CAD build for the part. Positions are in the model's coordinates, mm. Round coordinates to 2 decimals unless told otherwise and drop trailing zeros. Order: outer loops, then holes, each group sorted by start corner. A loop starts at its lowest first (then second) coordinate and runs counter-clockwise, first axis right, second up. Notation, with made-up numbers: (-32, -19) - (10, -19) arc R19 cw to (10, 14) - close; hole circle Ø3 at (6.5, 20.5). An arc over 180 degrees is marked (long way). Use one line per item in the form item = value. Start each with the question number.
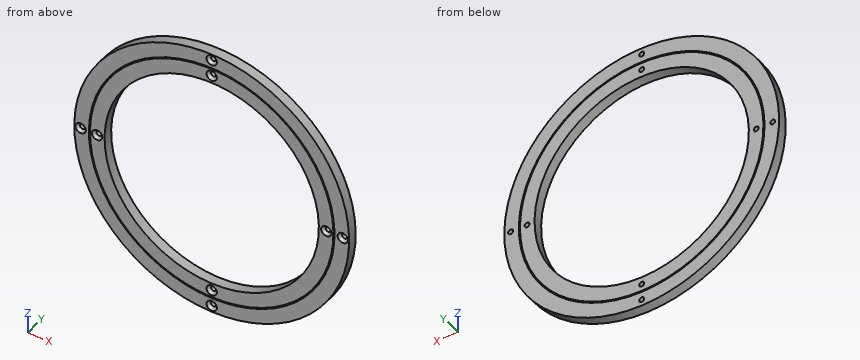
from build123d import *

# Parameters (mm, degrees)
CSK_FOR_M4_FLAT_HEAD_MACHINE_SCREW1_D           = 4.5
CSK_FOR_M4_FLAT_HEAD_MACHINE_SCREW1_CSINK_D     = 9.4
CSK_FOR_M4_FLAT_HEAD_MACHINE_SCREW1_CSINK_ANGLE = 90


with BuildPart() as part:
    # Sketch1 → Revolve1 (revolve)
    with BuildSketch(Plane.XY, mode=Mode.PRIVATE) as revolve1_sk:
        Polygon((-97.5, -4.5), (-97.5, 4.5), (-110.75, 4.5), (-110.75, 3.5), (-111.75, 3.5), (-111.75, 4.5), (-125, 4.5), (-125, -4.5), (-111.75, -4.5), (-111.75, -3.5), (-110.75, -3.5), (-110.75, -4.5), align=None)
    revolve(revolve1_sk.sketch.rotate(Axis((0, 0, 0), (0, 1, 0)), 270), axis=Axis((0, 0, 0), (0, 1, 0)))

    # CSK for M4 Flat Head Machine Screw1 (through all)
    with Locations(Plane(origin=(0, -4.5, 0), x_dir=(-1, 0, 0), z_dir=(0, -1, 0))):
        with Locations((-119.25, 0), (0, 104.25), (0, 119.25), (104.25, 0), (119.25, 0), (0, -104.25), (0, -119.25), (-104.25, 0)):
            CounterSinkHole(CSK_FOR_M4_FLAT_HEAD_MACHINE_SCREW1_D / 2, CSK_FOR_M4_FLAT_HEAD_MACHINE_SCREW1_CSINK_D / 2, counter_sink_angle=CSK_FOR_M4_FLAT_HEAD_MACHINE_SCREW1_CSINK_ANGLE)


solid = part.part
(1) Slice it at B-B (z = 29). Give the cut face in (x, y).
(2) Wall check: line 1 (Z direction, x = 73, y = -1.5); line 2 (X direction, y = 1.75, z = 27); line 3 (Z direction, x = -52, y = -0.75). Give the ranges that are in metal, low to high. Write a range as [from, to].
(3) Flat gauge pins, fed straight in: P1, Ø1.5, axis at y = -3, z = -99.5, coming from the -X side; P2, Ø4, axis at x = 27.5, y = 3, coming from the +Z side; P3, Ø6, axis at x = 119.25, z = 0, coming from the +Y side; P4, Ø2, axis at x = 87.5, y = 0.5, coming from the +Z side. Where does each tip first touch, or does it go through?
(4) Slice it at A-A (y = 1.5). Give the number of separate pieces and of enclosed holes in the cut face, and give its area (3 significant figures).
(5) Slice it at C-C (x = 79). Give the cut face in (y, z).
Results list:
q1.outline = (-121.59, -4.5) - (-107.92, -4.5) - (-107.92, -3.5) - (-106.89, -3.5) - (-106.89, -4.5) - (-93.09, -4.5) - (-93.09, 4.5) - (-106.89, 4.5) - (-106.89, 3.5) - (-107.92, 3.5) - (-107.92, 4.5) - (-121.59, 4.5) - close; (93.09, -4.5) - (106.89, -4.5) - (106.89, -3.5) - (107.92, -3.5) - (107.92, -4.5) - (121.59, -4.5) - (121.59, 4.5) - (107.92, 4.5) - (107.92, 3.5) - (106.89, 3.5) - (106.89, 4.5) - (93.09, 4.5) - close
q2.line_1 = [-101.47, -64.63], [64.63, 101.47]
q2.line_2 = [-122.05, -93.69], [93.69, 122.05]
q2.line_3 = [-113.67, -82.48], [82.48, 113.67]
q3.P1 = -76.64
q3.P2 = 122.37
q3.P3 = 4.5
q3.P4 = 90.24
q4.separate_pieces = 1
q4.enclosed_holes = 9
q4.area = 19,100 mm²
q5.outline = (-4.5, -96.87) - (4.5, -96.87) - (4.5, -79.04) - (3.5, -79.04) - (3.5, -77.62) - (4.5, -77.62) - (4.5, -57.14) - (-4.5, -57.14) - (-4.5, -77.62) - (-3.5, -77.62) - (-3.5, -79.04) - (-4.5, -79.04) - close; (-4.5, 57.14) - (4.5, 57.14) - (4.5, 77.62) - (3.5, 77.62) - (3.5, 79.04) - (4.5, 79.04) - (4.5, 96.87) - (-4.5, 96.87) - (-4.5, 79.04) - (-3.5, 79.04) - (-3.5, 77.62) - (-4.5, 77.62) - close
